```python
from build123d import *

# Parameters (mm, degrees)
SKETCH_1_R               = 20.5
EXTRUDE_1_DEPTH          = 8
CUT_EXTRUDE_1_DEPTH      = 31.074906484
CUT_EXTRUDE_1_DEPTH_BACK = 31.074906484
SKETCH_1_3_R             = 2.65
SKETCH_9_R               = 1
CUT_EXTRUDE_2_DEPTH      = 2.5
SKETCH_9_3_R             = 1
CUT_EXTRUDE_3_DEPTH      = 31.074906484
SKETCH_12_R              = 2.65
CUT_EXTRUDE_4_DEPTH      = 5


with BuildPart() as part:
    # Sketch 1 → Extrude 1 (new body)
    with BuildSketch(Plane.XY):
        Circle(SKETCH_1_R)
    extrude(amount=EXTRUDE_1_DEPTH)

    # Sketch 1_3 → Cut-Extrude 1 (cut, two sides: drawn at the far end of the back side and taken through both)
    with BuildSketch(Plane.XY.offset(-CUT_EXTRUDE_1_DEPTH_BACK)):
        Circle(SKETCH_1_3_R)
    extrude(amount=CUT_EXTRUDE_1_DEPTH + CUT_EXTRUDE_1_DEPTH_BACK, mode=Mode.SUBTRACT)

    # Sketch 9 → Cut-Extrude 2 (cut)
    # profile 1 of 2: a face of its own
    with BuildSketch(Plane.XY.offset(8)):
        with BuildLine():
            ThreePointArc((7.778174593, 7.778174593), (0, 11), (-7.778174593, 7.778174593))
            ThreePointArc((-7.778174593, 7.778174593), (-7.778174593, 3.535533906), (-3.535533906, 3.535533906))
            ThreePointArc((-3.535533906, 3.535533906), (0, 5), (3.535533906, 3.535533906))
            ThreePointArc((3.535533906, 3.535533906), (7.778174593, 3.535533906), (7.778174593, 7.778174593))
        make_face()
        with Locations((0, 8)):
            Circle(SKETCH_9_R, mode=Mode.SUBTRACT)
    # profile 2 of 2: a face of its own
    with BuildSketch(Plane.XY.offset(8)):
        with BuildLine():
            ThreePointArc((-7.778174593, -7.778174593), (-7.778174593, -3.535533906), (-3.535533906, -3.535533906))
            ThreePointArc((-3.535533906, -3.535533906), (0, -5), (3.535533906, -3.535533906))
            ThreePointArc((3.535533906, -3.535533906), (7.778174593, -3.535533906), (7.778174593, -7.778174593))
            ThreePointArc((7.778174593, -7.778174593), (0, -11), (-7.778174593, -7.778174593))
        make_face()
        with Locations((0, -8)):
            Circle(SKETCH_9_R, mode=Mode.SUBTRACT)
    extrude(amount=-CUT_EXTRUDE_2_DEPTH, mode=Mode.SUBTRACT)

    # Sketch 9_3 → Cut-Extrude 3 (cut, through all)
    with BuildSketch(Plane.XY.offset(8)):
        with Locations((0, 8)):
            Circle(SKETCH_9_3_R)
        with Locations((0, -8)):
            Circle(SKETCH_9_3_R)
    extrude(amount=-CUT_EXTRUDE_3_DEPTH, mode=Mode.SUBTRACT)

    # Sketch 12 → Cut-Extrude 4 (cut)
    with BuildSketch(Plane(origin=(0, 0, 0), x_dir=(-1, 0, 0), z_dir=(0, 0, -1))):
        with Locations((-12.5, 0)):
            Circle(SKETCH_12_R)
        with Locations((12.5, 0)):
            Circle(SKETCH_12_R)
    extrude(amount=-CUT_EXTRUDE_4_DEPTH, mode=Mode.SUBTRACT)


solid = part.part
```
Here's how the part is built. I have some questions about the finished solid (model axes, mm). A direction names the side the tool comes from. Coordinates: 2 decimals unless noted, no trailing zeros. Order: outer loops, then holes, each group sorted by start corner. A loop starts at its lowest first (then second) coordinate and runs counter-clockwise, first axis right, second up. Notation, with made-up numbers: M 51.5,16 L 84.5,16 A16 cw 84.5,33 Z; hole C 36.5,-6.75 d11. An arc over 180 degrees is marked long. Answer as a JSON object with one key per item and string values. Group by question number.
(1) Suppose I cut it at C-C, the plane x = 0. Please give me the cut outline in (y, z).
(2) For pin 1 (5 mm diameter, centred on x = 12.5, y = 0, fed in from -Z); pin 2 (1.5 mm diameter, centred on y = -12, z = 1, fed in from +X); pin 3 (1.8 mm diameter, centred on x = 0, y = -8, fed in from -Z); pin 4 (1.5 mm diameter, centred on x = 10.5, z = 6.5, fed in from +Y), each with a flat end and sliding along its axis, tell me the tip position at first contact or that it passes through.
(3) Suppose I cut it at B-B, the plane z = 7.25. Please give me the cut outline in (x, y), then the cut area to 3 significant figures.
(4) Which directions (+Z, -Z, +X, -X, +Y, -Y) give clear straight access to the entire face, cutting with the end or side of a thin tool? Please do faces 5 (the face through (0, 11, 7)), 6 (the face through (0, 9, 3)), 7 (the face through (-14.95, -1.01, 2.46)).
(5) Suppose I cut it at A-A, the plane y = 0. Please give me the cut outline in (x, z).
(6) Suppose I cut it at D-D, the plane z = 2.25. Please give me the cut outline in (x, y), then the cut area to 3 significant figures.
(7) If we mould it in two halves opening along Y, with no side actions, what happens to faces 1 (the face through (-4.444, -20.013, 3.944)), 2 (the face through (4, 0, 0)), 3 (the face through (7.73, 3.49, 6.77)), 4 (the face through (0, -7, 3))? For each: released by +Y, released by -Y, zero draft, split by the parting line, or undercut.
(8) I need wall thicknesses on probe 1 along Y at (x, z) = (0, 2.4); probe 2 along X at (y, z) = (-8.5, 2.5); probe 3 along Y at (x, z) = (-12, 4). Which ranges of each line are inside material? Lowest first, please.
Values found:
{
 "1": {"outline": "M -20.5,0 L -9,0 L -9,5.5 L -11,5.5 L -11,8 L -20.5,8 Z; M -7,0 L -2.65,0 L -2.65,8 L -5,8 L -5,5.5 L -7,5.5 Z; M 2.65,0 L 7,0 L 7,5.5 L 5,5.5 L 5,8 L 2.65,8 Z; M 9,0 L 20.5,0 L 20.5,8 L 11,8 L 11,5.5 L 9,5.5 Z"},
 "2": {"pin 1": "stops at z = 5", "pin 2": "stops at x = 17.14", "pin 3": "passes through", "pin 4": "stops at y = 18.03"},
 "3": {"outline": "C 0,0 d41; hole M -7.78,-7.78 A11 ccw 7.78,-7.78 A3 ccw 3.54,-3.54 A5 cw -3.54,-3.54 A3 ccw Z; hole M -7.78,7.78 A3 ccw -3.54,3.54 A5 cw 3.54,3.54 A3 ccw 7.78,7.78 A11 ccw Z; hole C 0,0 d5.3", "area": "1,090 mm^2"},
 "4": {"face 5": "+Z", "face 6": "+Z, -Z", "face 7": "-Z"},
 "5": {"outline": "M -20.5,0 L -15.15,0 L -15.15,5 L -9.85,5 L -9.85,0 L -2.65,0 L -2.65,8 L -20.5,8 Z; M 2.65,0 L 9.85,0 L 9.85,5 L 15.15,5 L 15.15,0 L 20.5,0 L 20.5,8 L 2.65,8 Z"},
 "6": {"outline": "C 0,0 d41; hole C -12.5,0 d5.3; hole C 0,0 d5.3; hole C 0,-8 d2; hole C 0,8 d2; hole C 12.5,0 d5.3", "area": "1,250 mm^2"},
 "7": {"face 1": "split by the parting line", "face 2": "zero draft", "face 3": "undercut", "face 4": "undercut"},
 "8": {"probe 1": "y = -20.5 to -9, -7 to -2.65, 2.65 to 7, 9 to 20.5", "probe 2": "x = -18.65 to -0.87, 0.87 to 18.65", "probe 3": "y = -16.62 to -2.6, 2.6 to 16.62"}
}
